from build123d import *

# Parameters (mm, degrees)
SKETCH1_W          = 13.1318
SKETCH1_H          = 29.718
EXTRUDE1_DEPTH     = 21.5392
SKETCH2_W          = 0.635
SKETCH2_H          = 29.718
CUT_EXTRUDE1_DEPTH = 14.732
SKETCH3_W          = 11.8618
SKETCH3_H          = 10.16
CUT_EXTRUDE2_DEPTH = 5.08
SKETCH5_W          = 1.778
SKETCH5_H          = 10.16
CUT_EXTRUDE3_DEPTH = 36.674017425
FILLET1_R          = 0.508
SKETCH7_W          = 7.493
SKETCH7_H          = 7.4168
EXTRUDE4_DEPTH     = 1.524
FILLET3_R          = 3.7338
SKETCH9_R          = 1.5621
CUT_EXTRUDE4_DEPTH = 1.524
SKETCH11_W         = 10.5918
SKETCH11_H         = 7.747
CUT_EXTRUDE5_DEPTH = 5.08
SKETCH12_W         = 10.5918
SKETCH12_H         = 9.271
CUT_EXTRUDE6_DEPTH = 5.08
SKETCH13_W         = 9.271
SKETCH13_H         = 7.62
EXTRUDE5_DEPTH     = 6.35
CHAMFER1_SIZE      = 1.27
SKETCH14_W         = 6.35
SKETCH14_H         = 7.62
CUT_EXTRUDE7_DEPTH = 3.048
SKETCH15_W         = 1.7272
SKETCH15_H         = 5.969
SKETCH15_W_2       = 5.715
SKETCH15_H_2       = 7.112
SKETCH15_R         = 0.127
CUT_EXTRUDE8_DEPTH = 5.08


with BuildPart() as part:
    # Sketch1 → Extrude1 (new body)
    with BuildSketch(Plane.XY):
        with Locations((6.5659, 14.859)):
            Rectangle(SKETCH1_W, SKETCH1_H)
    extrude(amount=EXTRUDE1_DEPTH)

    # Sketch2 → Cut-Extrude1 (cut)
    with BuildSketch(Plane.XY.offset(21.5392)):
        with Locations((0.3175, 14.859)):
            Rectangle(SKETCH2_W, SKETCH2_H)
        with Locations((12.8143, 14.859)):
            Rectangle(SKETCH2_W, SKETCH2_H)
    extrude(amount=-CUT_EXTRUDE1_DEPTH, mode=Mode.SUBTRACT)

    # Sketch3 → Cut-Extrude2 (cut)
    with BuildSketch(Plane.XY.offset(21.5392)):
        with Locations((6.5659, 15.621)):
            Rectangle(SKETCH3_W, SKETCH3_H)
    extrude(amount=-CUT_EXTRUDE2_DEPTH, mode=Mode.SUBTRACT)

    # Sketch5 → Cut-Extrude3 (cut, through all)
    with BuildSketch(Plane.XY.offset(6.8072)):
        with Locations((0.889, 15.621)):
            Rectangle(SKETCH5_W, SKETCH5_H)
        with Locations((12.2428, 15.621)):
            Rectangle(SKETCH5_W, SKETCH5_H)
    extrude(amount=CUT_EXTRUDE3_DEPTH, mode=Mode.SUBTRACT)

    # Fillet1
    fillet1_edges = [part.edges().sort_by_distance(p)[0] for p in [
        (0.635, 29.718, 14.1732),
        (0.635, 0, 14.1732),
        (12.4968, 0, 14.1732),
        (12.4968, 29.718, 14.1732),
        (12.4968, 20.701, 14.1732),
        (12.4968, 10.541, 14.1732),
        (0.635, 10.541, 14.1732),
        (0.635, 20.701, 14.1732),
    ]]
    fillet(fillet1_edges, radius=FILLET1_R)

    # Sketch7 → Extrude4 (add)
    with BuildSketch(Plane(origin=(0, 0, 0), x_dir=(-1, 0, 0), z_dir=(0, 0, -1))):
        with Locations((-6.5659, 33.4264)):
            Rectangle(SKETCH7_W, SKETCH7_H)
        with Locations((-6.5659, -3.7084)):
            Rectangle(SKETCH7_W, SKETCH7_H)
    extrude(amount=-EXTRUDE4_DEPTH)

    # Fillet3
    fillet3_edges = [part.edges().sort_by_distance(p)[0] for p in [
        (10.3124, 37.1348, 0.762),
        (2.8194, 37.1348, 0.762),
        (10.3124, -7.4168, 0.762),
        (2.8194, -7.4168, 0.762),
    ]]
    fillet(fillet3_edges, radius=FILLET3_R)

    # Sketch9 → Cut-Extrude4 (cut)
    with BuildSketch(Plane(origin=(0, 0, 0), x_dir=(-1, 0, 0), z_dir=(0, 0, -1))):
        with Locations((-6.5659, 33.401)):
            Circle(SKETCH9_R)
        with Locations((-6.5659, -3.683)):
            Circle(SKETCH9_R)
    extrude(amount=-CUT_EXTRUDE4_DEPTH, mode=Mode.SUBTRACT)

    # Sketch11 → Cut-Extrude5 (cut)
    with BuildSketch(Plane.XY.offset(21.5392)):
        with Locations((6.5659, 25.2095)):
            Rectangle(SKETCH11_W, SKETCH11_H)
    extrude(amount=-CUT_EXTRUDE5_DEPTH, mode=Mode.SUBTRACT)

    # Sketch12 → Cut-Extrude6 (cut)
    with BuildSketch(Plane.XY.offset(21.5392)):
        with Locations((6.5659, 5.2705)):
            Rectangle(SKETCH12_W, SKETCH12_H)
    extrude(amount=-CUT_EXTRUDE6_DEPTH, mode=Mode.SUBTRACT)

    # Sketch13 → Extrude5 (add)
    with BuildSketch(Plane.ZY):
        with Locations((4.6355, 14.859)):
            Rectangle(SKETCH13_W, SKETCH13_H)
    extrude(amount=EXTRUDE5_DEPTH)

    # Chamfer1
    chamfer1_edges = [part.edges().sort_by_distance(p)[0] for p in [
        (0, 14.859, 9.271),
    ]]
    chamfer(chamfer1_edges, length=CHAMFER1_SIZE)

    # Sketch14 → Cut-Extrude7 (cut)
    with BuildSketch(Plane(origin=(0, 0, 0), x_dir=(-1, 0, 0), z_dir=(0, 0, -1))):
        with Locations((3.175, 14.859)):
            Rectangle(SKETCH14_W, SKETCH14_H)
    extrude(amount=-CUT_EXTRUDE7_DEPTH, mode=Mode.SUBTRACT)

    # Sketch15 → Cut-Extrude8 (cut)
    # profile 1 of 2: a face of its own
    with BuildSketch(Plane.ZY.offset(6.35)):
        with Locations((3.4036, 24.1935)):
            Rectangle(SKETCH15_W, SKETCH15_H)
    # profile 2 of 2: a face of its own
    with BuildSketch(Plane.ZY.offset(6.35)):
        with Locations((6.1595, 14.859)):
            Rectangle(SKETCH15_W_2, SKETCH15_H_2)
        with Locations((7.76066841, 14.859)):
            Circle(SKETCH15_R, mode=Mode.SUBTRACT)
        with Locations((7.76066841, 17.399)):
            Circle(SKETCH15_R, mode=Mode.SUBTRACT)
        with Locations((7.76066841, 12.319)):
            Circle(SKETCH15_R, mode=Mode.SUBTRACT)
    extrude(amount=-CUT_EXTRUDE8_DEPTH, mode=Mode.SUBTRACT)


solid = part.part
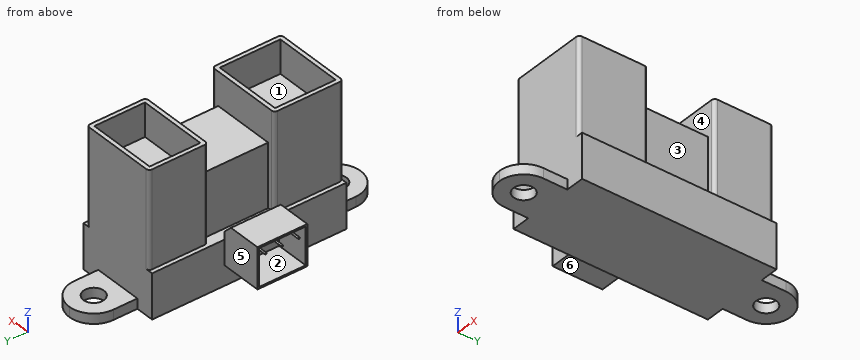
Verification items for the finished model (mm, model axes). Face numbers are marked on the shaded views. A direction names the side the tool comes from. Coordinates: 2 decimals unless noted, no trailing zeros. Order: outer loops, then holes, each group sorted by start corner. A loop starts at its lowest first (then second) coordinate and runs counter-clockwise, first axis right, second up. Notation, with made-up numbers: M 87,43 L 144,43 A13 cw 144,64 Z; hole C 0.25,75 d1. An arc over 180 degrees is marked long. Return JSON: item names as keys, results as strings.
1) Cross-section at D-D, the plane z = 3.75. Record the boundary of the cut face in (x, y) (3 decimals).
Answer list:
{"outline": "M -6.35,11.049 L 0,11.049 L 0,0 L 13.132,0 L 13.132,29.718 L 0,29.718 L 0,18.669 L -6.35,18.669 L -6.35,18.415 L -1.27,18.415 L -1.27,11.303 L -6.35,11.303 Z"}
2) Cross-section at A-A, the plane z = 18.5. Record the boundary of the cut face in (x, y) (3 decimals).
Answer list:
{"outline": "M 0.635,0.508 A0.508 ccw 1.143,0 L 11.989,0 A0.508 ccw 12.497,0.508 L 12.497,10.033 A0.508 ccw 11.989,10.541 L 1.143,10.541 A0.508 ccw 0.635,10.033 Z; M 0.635,21.209 A0.508 ccw 1.143,20.701 L 11.989,20.701 A0.508 ccw 12.497,21.209 L 12.497,29.21 A0.508 ccw 11.989,29.718 L 1.143,29.718 A0.508 ccw 0.635,29.21 Z; hole M 1.27,0.635 L 11.862,0.635 L 11.862,9.906 L 1.27,9.906 Z; hole M 1.27,21.336 L 11.862,21.336 L 11.862,29.083 L 1.27,29.083 Z"}
3) Cross-section at C-C, the plane y = 2. Record the boundary of the cut face in (x, z) (3 decimals).
Answer list:
{"outline": "M 0,0 L 13.132,0 L 13.132,6.807 L 12.497,6.807 L 12.497,21.539 L 11.862,21.539 L 11.862,16.459 L 1.27,16.459 L 1.27,21.539 L 0.635,21.539 L 0.635,6.807 L 0,6.807 Z"}
4) Release check for a two-part mould opening along Y. For the marked faces 4, 5 and 6 record: +Y half, -Y half, draft (parallel to the pull), parting line (faces both ways), or undercut.
Answer list:
{"face 4": "undercut", "face 5": "+Y half", "face 6": "draft"}
5) Thickness scan on L1, parallel to Y at x = 6.75, z = 17.75 (3 decimals); L2, parallel to Y at x = -3.5, z = 8.5 (3 decimals); L3, parallel to X at y = 5.5, z = 16.75 (3 decimals). Record the ranges inside material, lowest first. Write a range as [from, to].
Answer list:
{"L1": "[0, 0.635], [9.906, 10.541], [20.701, 21.336], [29.083, 29.718]", "L2": "[11.049, 11.303], [18.415, 18.669]", "L3": "[0.635, 1.27], [11.862, 12.497]"}
6) Gauge pin test, flat ends, axial feed: pin 1 (4 mm diameter, centred on y = 27, z = 20, fed in from -X) (3 decimals); pin 2 (2.5 mm diameter, centred on y = 25.5, z = 19.5, fed in from +X); pin 3 (5.5 mm diameter, centred on x = -4.5, z = 6.5, fed in from -Y). Record the tip position at first contact, or that the pin passes through.
Answer list:
{"pin 1": "x = 0.635", "pin 2": "x = 12.5", "pin 3": "y = 11.05"}
7) Access from +Z, -Z, +X, -X, +Y, -Y to the whole of each face (thin tool, end or side, straight path). Record for the marked faces 1, 2 and 3.
Answer list:
{"face 1": "+Z", "face 2": "-X", "face 3": "+Z, +X"}
8) Cross-section at B-B, the plane x = -5. Record the boundary of the cut face in (y, z) (3 decimals), and give its area (3 significant figures).
Answer list:
{"outline": "M 11.049,3.048 L 18.669,3.048 L 18.669,9.271 L 11.049,9.271 Z; C 12.319,7.761 d0.254; C 14.859,7.761 d0.254; C 17.399,7.761 d0.254; hole M 11.303,3.302 L 18.415,3.302 L 18.415,9.017 L 11.303,9.017 Z", "area": "6.93 mm2"}
